Here's the drawing with two shaded views (mm, measured from the low corner). I have some questions. A direction names the side the tool comes from. Round coordinates to 2 decimals unless told otherwise and drop trailing zeros. Loops run counter-clockwise (first coordinate to the right, second up) from the corner with the lowest first, then second, coordinate; pieces in that order, holes last.
(1) Will these pins go through, and if not, where does the flat tip stop? pin 1 Ø1 at (x, z) = (3, 2.5) entering from +Y; pin 2 Ø1.3 at (y, z) = (5, 2.5) entering from -X; pin 3 Ø1.3 at (x, z) = (8.5, 3.5) entering from -Y.
(2) If I drill on line 1 along Y through (x, z) = (12.5, 4.75); line 2 along Z through (x, y) = (2.5, 1); line 3 along X through (y, z) = (4, 2) (1 decimal), over which ranges is the centre line in solid material (lowest first)?
(3) Which directions (+Z, -Z, +X, -X, +Y, -Y) give clear straight access to the entire face, cutting with the end or side of a thin tool? Please do the marked faces 1, 2, 3, 4 and 5.
(4) I want a section at C-C on z = 3.75. Write out the boundary of the cut face in (x, y) (1 decimal).
(5) I want a section at D-D on y = 8.25. Write out the boundary of the cut face in (x, z) (1 decimal), plus the area to 3 significant figures.
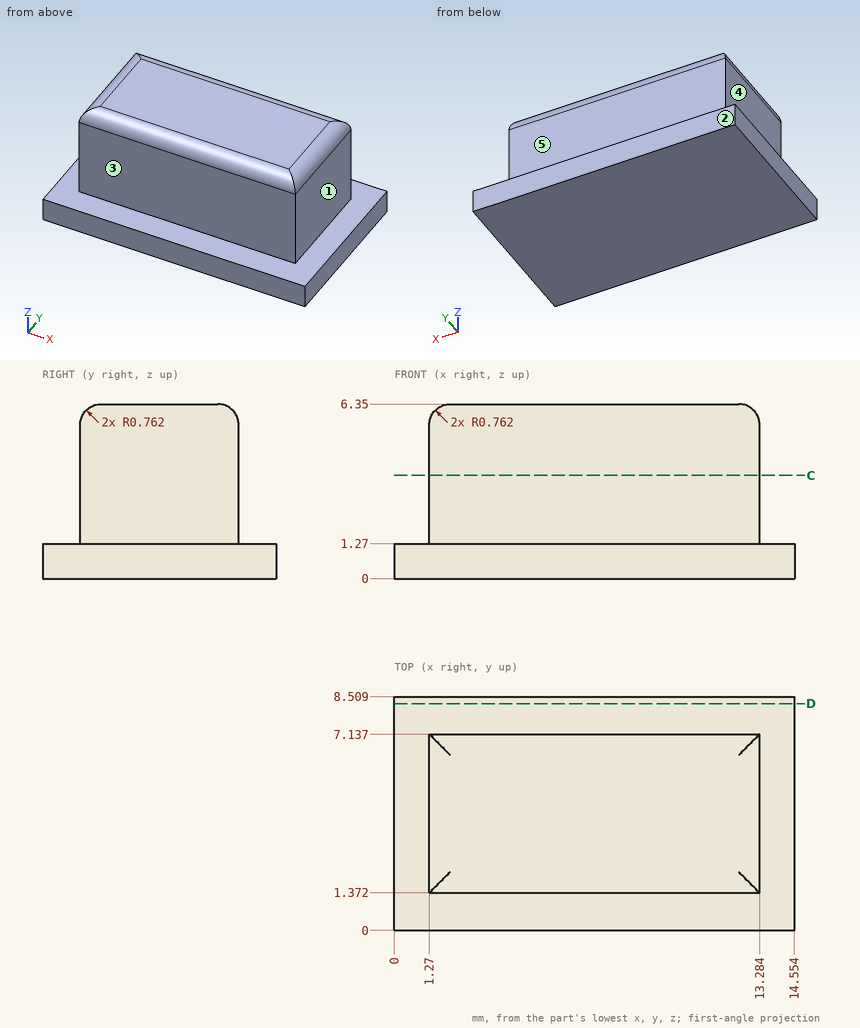
Filled sheet:
1. pin 1: stops at y = 7.14
1. pin 2: stops at x = 1.27
1. pin 3: stops at y = 1.37
2. line 1: y = 1.37 to 7.14
2. line 2: z = 0 to 1.27
2. line 3: x = 1.3 to 13.3
3. face 1: +Z, +X, +Y, -Y
3. face 2: +Z, -Z, +X, -X, +Y
3. face 3: +Z, +X, -X, -Y
3. face 4: +Z, -X, +Y, -Y
3. face 5: +Z, +X, -X, +Y
4. outline: (1.3, 1.4) - (13.3, 1.4) - (13.3, 7.1) - (1.3, 7.1) - close
5. outline: (0, 0) - (14.6, 0) - (14.6, 1.3) - (0, 1.3) - close
5. area: 18.5 mm2
